Autodesk Inventor part; units mm, degrees
ref_plane "YZ Plane" through (0, 0, 0) normal (1, 0, 0) x (0, 1, 0)
ref_plane "XZ Plane" through (0, 0, 0) normal (0, 1, 0) x (-1, 0, 0)
ref_plane "XY Plane" through (0, 0, 0) normal (0, 0, 1) x (1, 0, 0)
sketch "스케치3" plane through (0, 0, 0) normal (0, 1, 0) x (-1, 0, 0)
  line L0 (35.5919, -14.7426) -> (14.7426, -35.5919)
  line L1 (14.7426, -35.5919) -> (-14.7426, -35.5919)
  line L2 (-14.7426, -35.5919) -> (-35.5919, -14.7426)
  line L3 (-35.5919, -14.7426) -> (-35.5919, 14.7426)
  line L4 (-35.5919, 14.7426) -> (-14.7426, 35.5919)
  line L5 (-14.7426, 35.5919) -> (14.7426, 35.5919)
  line L6 (14.7426, 35.5919) -> (35.5919, 14.7426)
  line L7 (35.5919, 14.7426) -> (35.5919, -14.7426)
  line L8 (32.5919, -13.5) -> (13.5, -32.5919)
  line L9 (13.5, -32.5919) -> (-13.5, -32.5919)
  line L10 (-13.5, -32.5919) -> (-32.5919, -13.5)
  line L11 (-32.5919, -13.5) -> (-32.5919, 13.5)
  line L12 (-32.5919, 13.5) -> (-13.5, 32.5919)
  line L13 (-13.5, 32.5919) -> (13.5, 32.5919)
  line L14 (13.5, 32.5919) -> (32.5919, 13.5)
  line L15 (32.5919, 13.5) -> (32.5919, -13.5)
  point P0 (0, 0)
  point P1 (0, 0)
  point P2 (0, 0)
  point P3 (0, 0)
  dimension "d43" = 27
  dimension "d44" = 3
extrude "돌출2" add sketch "스케치3" along normal blind 4.4 contours L0 L1 L2 L3 L4 L5 L6 L7 | L8 L9 L10 L11 L12 L13 L14 L15
sketch "스케치4" plane through (0, 4.4, 0) normal (0, 1, 0) x (1, 0, 0)
  line L0 (13.5, -32.5919) -> (-13.5, -32.5919)
  line L1 (-13.5, -32.5919) -> (-32.5919, -13.5)
  line L2 (-32.5919, -13.5) -> (-32.5919, 13.5)
  line L3 (-32.5919, 13.5) -> (-13.5, 32.5919)
  line L4 (-13.5, 32.5919) -> (13.5, 32.5919)
  line L5 (13.5, 32.5919) -> (32.5919, 13.5)
  line L6 (32.5919, 13.5) -> (32.5919, -13.5)
  line L7 (32.5919, -13.5) -> (13.5, -32.5919)
  line L8 (-14.2456, 34.3919) -> (14.2456, 34.3919)
  line L9 (14.2456, 34.3919) -> (34.3919, 14.2456)
  line L10 (34.3919, 14.2456) -> (34.3919, -14.2456)
  line L11 (34.3919, -14.2456) -> (14.2456, -34.3919)
  line L12 (14.2456, -34.3919) -> (-14.2456, -34.3919)
  line L13 (-14.2456, -34.3919) -> (-34.3919, -14.2456)
  line L14 (-34.3919, -14.2456) -> (-34.3919, 14.2456)
  line L15 (-34.3919, 14.2456) -> (-14.2456, 34.3919)
  line L16 (-13.4172, 32.3919) -> (13.4172, 32.3919)
  line L17 (13.4172, 32.3919) -> (32.3919, 13.4172)
  line L18 (32.3919, 13.4172) -> (32.3919, -13.4172)
  line L19 (32.3919, -13.4172) -> (13.4172, -32.3919)
  line L20 (13.4172, -32.3919) -> (-13.4172, -32.3919)
  line L21 (-13.4172, -32.3919) -> (-32.3919, -13.4172)
  line L22 (-32.3919, -13.4172) -> (-32.3919, 13.4172)
  line L23 (-32.3919, 13.4172) -> (-13.4172, 32.3919)
  point P0 (0, 0)
  point P1 (0, 0)
  point P2 (0, 0)
  point P3 (0, 0)
  dimension "d7" = 27
  dimension "d42" = 1.8
  dimension "d45" = 0.2
extrude "돌출3" cut sketch "스케치4" against normal blind 1.2 contours L0 L1 L2 L3 L4 L5 L6 L7 | L8 L9 L10 L11 L12 L13 L14 L15 | L16 L17 L18 L19 L20 L21 L22 L23
sketch "스케치5" plane through (0, 0, 0) normal (0, -1, 0) x (1, 0, 0)
  line L0 (10, 2.5) -> (20, 2.5)
  line L1 (20, 2.5) -> (20, -2.5)
  line L2 (20, -2.5) -> (10, -2.5)
  line L3 (10, -2.5) -> (10, 2.5)
  line L4 (10, 2.5) -> (20, -2.5) construction
  line L5 (20, 2.5) -> (10, -2.5) construction
  line L6 (-20, 2.5) -> (-10, 2.5)
  line L7 (-10, 2.5) -> (-10, -2.5)
  line L8 (-10, -2.5) -> (-20, -2.5)
  line L9 (-20, -2.5) -> (-20, 2.5)
  line L10 (-20, 2.5) -> (-10, -2.5) construction
  line L11 (-10, 2.5) -> (-20, -2.5) construction
  point P0 (0, 0)
  point P1 (15, 0)
  point P2 (-15, 0)
  dimension "d11" = 10
  dimension "d12" = 5
  dimension "d13" = 10
  dimension "d16" = 30
extrude "돌출4" add sketch "스케치5" along normal blind 10
sketch "스케치6" plane through (-10, 0, -2.5) normal (0, 0, -1) x (-1, 0, 0)
  circle A0 centre (5, -10) radius 5
  circle A1 centre (-25, -10) radius 5
  line L0 (-20, -10) -> (-30, -10)
  line L1 (10, -10) -> (0, -10)
  point P0 (-10, 0)
  dimension "d23" = 10
  dimension "d24" = 10
extrude "돌출5" add sketch "스케치6" against normal blind 5
sketch "스케치7" plane through (-10, 0, -2.5) normal (0, 0, -1) x (-1, 0, 0)
  circle A0 centre (5, -10) radius 1.25
  line L0 (10, 0) -> (10, -10)
  line L1 (0, 0) -> (10, 0)
  line L2 (4.7788, 0) -> (0, 0)
  circle A1 centre (-25, -10) radius 1.25
  point P0 (-10, 0)
  dimension "d27" = 2.5
  dimension "d28" = 5
  dimension "d31" = 30
extrude "돌출6" cut sketch "스케치7" against normal blind 5
sketch "스케치8" plane through (0, 0, 0) normal (0, -1, 0) x (1, 0, 0)
  circle A0 centre (0, -17.3205) radius 1.25
  line L0 (-10, 2.5) -> (-10, -2.5)
  point P0 (0, 0)
  point P1 (-10, 0)
  dimension "d38" = 2.5
  dimension "d39" = 17.3205
sketch "스케치9" plane through (0, 3.2, 0) normal (0, 1, 0) x (1, 0, 0)
  line L0 (-13.4172, 32.3919) -> (13.4172, 32.3919)
  line L1 (13.4172, 32.3919) -> (32.3919, 13.4172)
  line L2 (32.3919, 13.4172) -> (32.3919, -13.4172)
  line L3 (32.3919, -13.4172) -> (13.4172, -32.3919)
  line L4 (13.4172, -32.3919) -> (-13.4172, -32.3919)
  line L5 (-13.4172, -32.3919) -> (-32.3919, -13.4172)
  line L6 (-32.3919, -13.4172) -> (-32.3919, 13.4172)
  line L7 (-32.3919, 13.4172) -> (-13.4172, 32.3919)
  line L8 (-14.2456, 34.3919) -> (14.2456, 34.3919)
  line L9 (-12.1745, 29.3919) -> (12.1745, 29.3919)
  line L10 (12.1745, 29.3919) -> (29.3919, 12.1745)
  line L11 (29.3919, 12.1745) -> (29.3919, -12.1745)
  line L12 (29.3919, -12.1745) -> (12.1745, -29.3919)
  line L13 (12.1745, -29.3919) -> (-12.1745, -29.3919)
  line L14 (-12.1745, -29.3919) -> (-29.3919, -12.1745)
  line L15 (-29.3919, -12.1745) -> (-29.3919, 12.1745)
  line L16 (-29.3919, 12.1745) -> (-12.1745, 29.3919)
  point P0 (0, 0)
  point P1 (0, 0)
  point P2 (0, 0)
  dimension "d46" = 2
  dimension "d47" = 3
extrude "돌출8" add sketch "스케치9" along normal blind 0.6 contours L0 L1 L2 L3 L4 L5 L6 L7 | L9 L10 L11 L12 L13 L14 L15 L16
fillet "모깎기1" radius 1.2 16 edges at (-35.5919, 4.4, 0) (-25.1673, 4.4, 25.1673) (0, 4.4, 35.5919) (25.1673, 4.4, 25.1673) (35.5919, 4.4, 0) (25.1673, 4.4, -25.1673) (0, 4.4, -35.5919) (-25.1673, 4.4, -25.1673) (25.1673, 0, 25.1673) (0, 0, 35.5919) (-25.1673, 0, 25.1673) (-35.5919, 0, 0) (-25.1673, 0, -25.1673) (0, 0, -35.5919) (25.1673, 0, -25.1673) (35.5919, 0, 0)
sketch "스케치10" plane through (0, 0, 0) normal (0, -1, 0) x (1, 0, 0)
  line L0 (-20, 2.5) -> (-10, 2.5)
  line L1 (-10, -2.5) -> (-20, -2.5)
  line L2 (-20, 2.5) -> (-19, 2.5)
  line L3 (-19, 2.5) -> (-19, -2.5)
  line L4 (-19, -2.5) -> (-20, -2.5)
  line L5 (-20, -2.5) -> (-20, 2.5)
  line L6 (20, -2.5) -> (10, -2.5)
  line L7 (10, 2.5) -> (20, 2.5)
  line L8 (20, -2.5) -> (19, -2.5)
  line L9 (19, -2.5) -> (19, 2.5)
  line L10 (19, 2.5) -> (20, 2.5)
  line L11 (20, 2.5) -> (20, -2.5)
  point P0 (0, 0)
  dimension "d54" = 1
  dimension "d55" = 1
extrude "돌출9" cut sketch "스케치10" along normal blind 15
extrude "돌출10" cut sketch "스케치8" against normal blind 5
equation "\"d55\" = d54"
properties part number "OV-PAM_top_2"
The model under review builds one solid part; all positions refer to its coordinate system, in mm. A direction names the side the tool comes from. Round coordinates to 2 decimals unless told otherwise and drop trailing zeros. Return JSON: item names as keys, results as strings.
1. Insertion check: P1, Ø3, axis at x = 14, y = -9, coming from the -Z side; P2, Ø1.5, axis at x = 0, z = -17.32, coming from the +Y side; P3, Ø4, axis at y = -7, z = -0.5, coming from the -X side; P4, Ø4, axis at y = -7, z = -0.5, coming from the +X side. Each pin has a flat end and moves straight along its axis. Give the tip position at first contact, or say it passes through.
Answer block:
{"P1": "stops at z = -2.5", "P2": "passes through", "P3": "stops at x = -19", "P4": "stops at x = 19"}
2. For L1, parallel to Z at x = 12.5, y = 3.25; L2, parallel to Y at x = 15, z = 0; L3, parallel to X at y = 3.5, z = -17.5, list the stretches that pass through material, from the lowest coordinate up. Write a range as [from, to].
Answer block:
{"L1": "z = [-35.59, -34.39], [-32.39, 32.39], [34.39, 35.59]", "L2": "y = [-15, -11.25], [-8.75, 3.8]", "L3": "x = [-32.78, -31.14], [-28.31, -1.24], [1.24, 28.31], [31.14, 32.78]"}
3. For faces 4 (the face through (14, -7, 2.5)), 5 (the face through (-24.766, 0.342, -25.058)), 6 (the face through (-25.021, 2.186, 25.313)), 7 (the face through (-22.77, 3.5, 23.04)), 8 (the face through (-10, -5, 0)), list the 3-axis set-ups (+Z, -Z, +X, -X, +Y, -Y) from which the entire face can be reached by the end or side of a thin tool; tool diameter is ignored.
Answer block:
{"face 4": "+Z, +X, -X, -Y", "face 5": "-Z, -X, -Y", "face 6": "+Z, -X, +Y, -Y", "face 7": "+Y", "face 8": "+Z, -Z, -Y"}
4. The part is to be moulded in two halves that separate along X. For faces 1 (the face through (16.25, -9.95, -0.04)), 2 (the face through (-35.592, 2, 0)), 3 (the face through (24.766, 0.342, 25.058)), say which applies: +X half, -X half, draft (parallel to the pull), parting line (faces both ways), or undercut.
Answer block:
{"face 1": "undercut", "face 2": "-X half", "face 3": "+X half"}
